```python
from build123d import *

# Parameters (mm, degrees)
CUT_EXTRUDE_THIN1_DEPTH = 14.266499161


with BuildPart() as part:
    # Sketch1 → Revolve1 (revolve)
    with BuildSketch(Plane.XY, mode=Mode.PRIVATE) as revolve1_sk:
        Polygon((-12, 2.8), (12, 2.8), (12, 3.5992), (11.140481626, 4), (-11.140481626, 4), (-12, 3.5992), align=None)
    revolve(revolve1_sk.sketch.rotate(Axis((-12, 0, 0), (1, 0, 0)), 90), axis=Axis((-12, 0, 0), (1, 0, 0)))

    # Sketch2 → Cut-Extrude-Thin1 (cut, through all)
    with BuildSketch(Plane.XY):
        Polygon((-12, -0.125), (-7.425623157, -0.125), (-7.104084127, 1.075), (7.104084127, 1.075), (7.425623157, -0.125), (12, -0.125), (12, 0.125), (7.617454904, 0.125), (7.295915873, 1.325), (-7.295915873, 1.325), (-7.617454904, 0.125), (-12, 0.125), align=None)
    extrude(amount=CUT_EXTRUDE_THIN1_DEPTH, mode=Mode.SUBTRACT)


solid = part.part
```
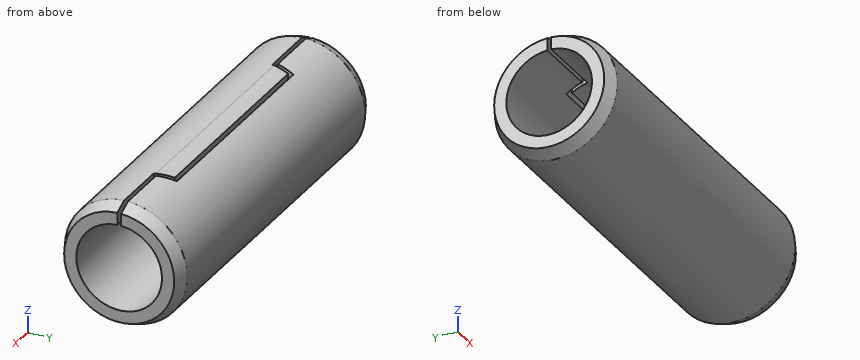
For this review, take the finished solid that the model builds, in its own axes (mm). Round coordinates to 2 decimals unless told otherwise and drop trailing zeros. Write each loop counter-clockwise with the first axis right and the second up, starting at its lowest first coordinate (ties: lowest second). Pieces come first, ordered by that corner, then holes. Notation, with made-up numbers: (10, -4) - (58, -4) arc R16 ccw to (58, 27) - close; hole circle Ø8 at (61, -31). An arc over 180 degrees is marked (long way). Answer as a JSON object with one key per item and string values.
1. We need section C-C on x = -8. Give the boundary of the cut face in (y, z) (3 decimals).
Response values:
{"outline": "(-0.125, 2.797) - (-0.125, 3.998) arc R4 ccw (long way) to (0.125, 3.998) - (0.125, 2.797) arc R2.8 cw (long way) to start"}
2. For pin 1 Ø1.5 at (x, z) = (-6, -3) entering from +Y; pin 2 Ø1.3 at (x, z) = (-9, 3.5) entering from +Y; pin 3 Ø0.6 at (x, z) = (9.5, 3.5) entering from -Y, all flat-tipped, find the tip position at first contact; note any pin that passes through.
Response values:
{"pin 1": "stops at y = 3.31", "pin 2": "stops at y = 2.81", "pin 3": "stops at y = -2.4"}
3. To check wall thickness, follow line 1 along Y through (x, z) = (3, 0); line 2 along Z through (x, y) = (1.5, 0.5) (3 decimals); line 3 along Y through (x, z) = (-5.5, 1.5). State the ranges of each line that lie inside material, in increasing order.
Response values:
{"line 1": "y = -4 to -2.8, 2.8 to 4", "line 2": "z = -3.969 to -2.755, 2.755 to 3.969", "line 3": "y = -3.71 to -2.36, 2.36 to 3.71"}
4. We need section B-B on x = 0.25. Give the boundary of the cut face in (y, z) (3 decimals), then the cut area to 3 significant figures.
Response values:
{"outline": "(1.075, 2.585) - (1.075, 3.853) arc R4 ccw (long way) to (1.325, 3.774) - (1.325, 2.467) arc R2.8 cw (long way) to start", "area": "25.3 mm2"}
5. We need section A-A on z = 0. Give the boundary of the cut face in (x, y).
Response values:
{"outline": "(-12, -3.6) - (-11.14, -4) - (11.14, -4) - (12, -3.6) - (12, -2.8) - (-12, -2.8) - close; (-12, 2.8) - (12, 2.8) - (12, 3.6) - (11.14, 4) - (-11.14, 4) - (-12, 3.6) - close"}
